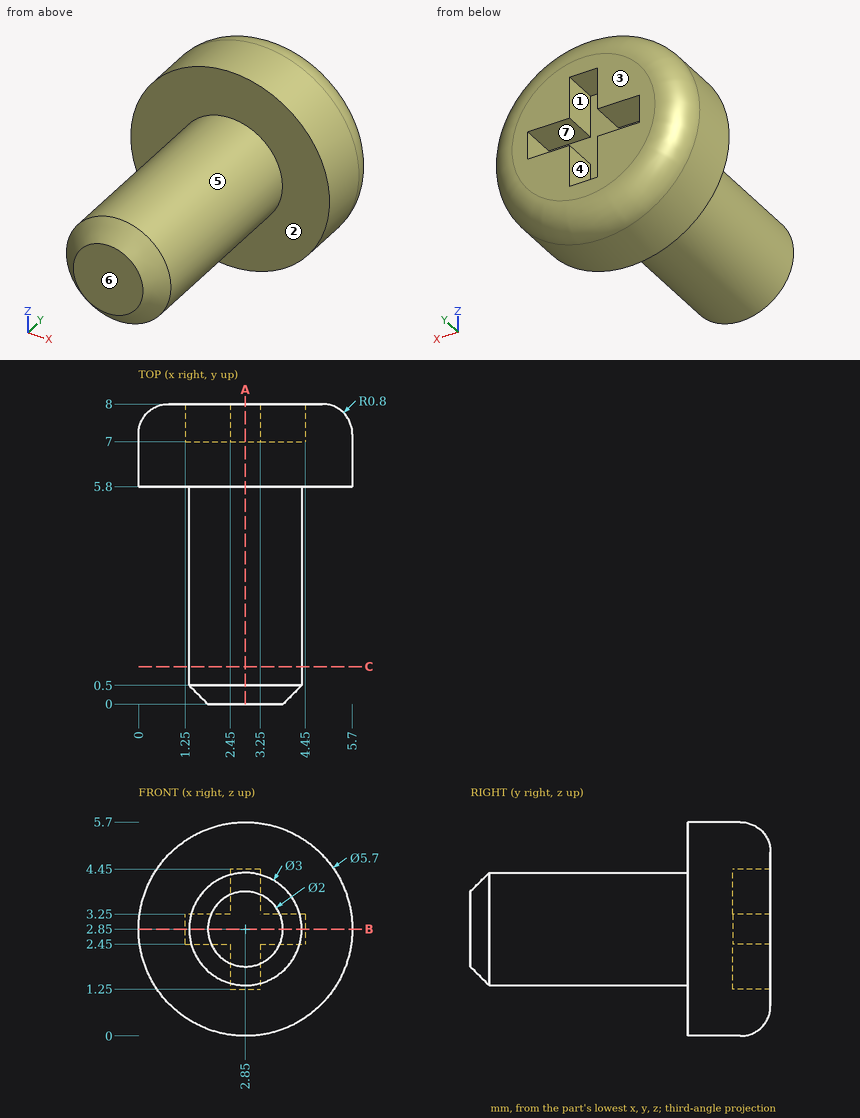
Design review of the part shown in the three views and the two pictorial views. Dimensions are in mm from the part's minimum x, y and z. A direction names the side the tool comes from. Give positions to 0.01 mm unless a question says otherwise; leave off trailing zeros. Write each loop counter-clockwise with the first axis right and the second up, starting at its lowest first coordinate (ties: lowest second). Pieces come first, ordered by that corner, then holes. Notation, with made-up numbers: M -34,19 L 23,19 A15 cw 23,33 Z; hole C 34,35 d1. An arc over 180 degrees is marked long. Return JSON: item names as keys, results as strings. Group by question number.
Item 1: Take a section at A-A (x = 2.85). Give the boundary of the cut face in (y, z), plus the area to 3 significant figures.
Item 2: Clearance check with flat-ended pins moving along their axes: pin 1 Ø2 at (y, z) = (2.5, 1.5) entering from +X; pin 2 Ø1.1 at (y, z) = (7.5, 1.5) entering from -X; pin 3 Ø1.1 at (y, z) = (7.5, 4) entering from +X. State where each tip first meets the part, or that it passes through.
Item 3: Take a section at C-C (y = 1). Give the boundary of the cut face in (x, z), plus the area to 3 significant figures.
Item 4: Wall thickness on line 1 along Y through (x, z) = (3.6, 2.5); line 2 along Y through (x, z) = (4.25, 4.1); line 3 along X through (y, z) = (1.5, 3.2): over which ranges is each line inside the solid? List them lowest first.
Item 5: Tool access review of the marked faces 1, 2 and 3: name each direction out of +Z, -Z, +X, -X, +Y, -Y from which nothing blocks a thin tool from reaching the whole face with its end or side.
Item 6: Take a section at B-B (z = 2.85). Give the boundary of the cut face in (x, y).
Item 7: The part is to be moulded in two halves that separate along Z. For the marked faces 4, 5, 6 and 7, say which applies: pulls with the +Z half, pulls with the -Z half, needs draft (parallel to the pull), parting line crosses it, or undercut.
Return value:
{
 "1": {"outline": "M 0,1.85 L 0.5,1.35 L 5.8,1.35 L 5.8,0 L 7.2,0 A0.8 ccw 8,0.8 L 8,1.25 L 7,1.25 L 7,4.45 L 8,4.45 L 8,4.9 A0.8 ccw 7.2,5.7 L 5.8,5.7 L 5.8,4.35 L 0.5,4.35 L 0,3.85 Z", "area": "26.2 mm2"},
 "2": {"pin 1": "stops at x = 4.31", "pin 2": "stops at x = 0.13", "pin 3": "stops at x = 5.62"},
 "3": {"outline": "C 2.85,2.85 d3", "area": "7.07 mm2"},
 "4": {"line 1": "y = 0 to 7", "line 2": "y = 5.8 to 8", "line 3": "x = 1.39 to 4.31"},
 "5": {"face 1": "+Y", "face 2": "-Y", "face 3": "+Z, -Z, +X, -X, +Y"},
 "6": {"outline": "M 0,5.8 L 1.35,5.8 L 1.35,0.5 L 1.85,0 L 3.85,0 L 4.35,0.5 L 4.35,5.8 L 5.7,5.8 L 5.7,7.2 A0.8 ccw 4.9,8 L 4.45,8 L 4.45,7 L 1.25,7 L 1.25,8 L 0.8,8 A0.8 ccw 0,7.2 Z"},
 "7": {"face 4": "undercut", "face 5": "parting line crosses it", "face 6": "needs draft", "face 7": "undercut"}
}
